Design review of the part built by this model. Coordinates are the model's own, in mm. Face numbers are marked on the shaded views. A direction names the side the tool comes from. Give positions to 0.01 mm unless a question says otherwise; leave off trailing zeros. Loops run counter-clockwise (first coordinate to the right, second up) from the corner with the lowest first, then second, coordinate; pieces in that order, holes last. Notation, with made-up numbers: M 64,-0.5 L 116,-0.5 A26 ccw 116,35.5 Z; hole C 48,-25 d10. An arc over 180 degrees is marked long. Use a Markdown table: item, result. Add a question column.
(1) For the marked faces 1, 2 and 3, list the 3-axis set-ups (+Z, -Z, +X, -X, +Y, -Y) from which the entire face can be reached by the end or side of a thin tool; tool diameter is ignored.
(2) Add section C-C, the plane x = 19.25. Give the boundary of the cut face in (y, z), then the cut area to 3 significant figures.
(3) Add section D-D, the plane z = 48.5. Give the boundary of the cut face in (x, y), then the cut area to 3 significant figures.
(4) Add section A-A, the plane y = -33. Give the boundary of the cut face in (x, z), then the cut area to 3 significant figures.
(5) Insertion check: pin 1 Ø12 at (x, z) = (23.5, 13.5) entering from +Y; pin 2 Ø8 at (x, y) = (19.5, -40.5) entering from -Z; pin 3 Ø4 at (x, y) = (26, -29.5) entering from -Z; pin 4 Ø1.8 at (x, z) = (33.7, 18.8) entering from +Y. Each pin has a flat end and moves straight along its axis. Give the tip position at first contact, or say it passes through.
(6) Add section B-B, the plane z = 18.8. Give the boundary of the cut face in (x, y), then the cut area to 3 significant figures.
(7) Draft analysis for pull direction Z (two halves, no side actions). For the marked faces 4 and 5, state which applies: pulls with the +Z half, pulls with the -Z half, needs draft (parallel to the pull), parting line crosses it, or undercut.
(8) For probe 1 along X at (y, z) = (-27.1, 18.8); probe 2 along Z at (x, y) = (33.7, -27.15); probe 3 along Y at (x, z) = (32, 45), list the stretches that pass through material, from the lowest coordinate up.
```python
from build123d import *

# Parameters (mm, degrees)
SKETCH009_W             = 20
SKETCH009_H             = 35
SKETCH009_R             = 1.5
PAD007_DEPTH            = 2
SKETCH010_R             = 10
PAD008_DEPTH            = 15
SKETCH011_R             = 1.5
PAD009_DEPTH            = 1
SKETCH012_W             = 10
SKETCH012_H             = 2.3
PAD010_DEPTH            = 6
SKETCH013_W             = 10
SKETCH013_H             = 2.3
PAD011_DEPTH            = 11
BODY002_PLACEMENT_ANGLE = 180


with BuildPart() as part:
    # Sketch009 → Pad007 (new body)
    with BuildSketch(Plane.XZ):
        Rectangle(SKETCH009_W, SKETCH009_H)
        with Locations((7.7, 15.2)):
            Circle(SKETCH009_R, mode=Mode.SUBTRACT)
        with Locations((-7.7, 15.2)):
            Circle(SKETCH009_R, mode=Mode.SUBTRACT)
    extrude(amount=PAD007_DEPTH)

    # Sketch010 (on Face8 of Pad007) → Pad008 (join)
    with BuildSketch(Plane.XZ.offset(2)):
        with Locations((0, -6)):
            Circle(SKETCH010_R)
    extrude(amount=PAD008_DEPTH)

    # Sketch011 (on Face4 of Pad008) → Pad009 (join)
    with BuildSketch(Plane(origin=(0, 0, 0), x_dir=(1, 0, 0), z_dir=(0, 1, 0))):
        with Locations((0, 7.5)):
            Circle(SKETCH011_R)
    extrude(amount=PAD009_DEPTH)

    # Sketch012 (on Face5 of Pad009) → Pad010 (join)
    with BuildSketch(Plane.XZ.offset(2)):
        with Locations((0, 15.35)):
            Rectangle(SKETCH012_W, SKETCH012_H)
    extrude(amount=PAD010_DEPTH)

    # Sketch013 (on Face13 of Pad010) → Pad011 (join)
    with BuildSketch(Plane(origin=(0, 0, 16.5), x_dir=(-1, 0, 0), z_dir=(0, 0, 1))):
        with Locations((0, 6.85)):
            Rectangle(SKETCH013_W, SKETCH013_H)
    extrude(amount=PAD011_DEPTH)


with BuildPart() as part_1:
    # Body002 placement: moved
    add(part.part.moved(Location((26, -26, 34))).rotate(Axis((26, -26, 34), (0, 1, 0)), BODY002_PLACEMENT_ANGLE))


solid = part_1.part
```
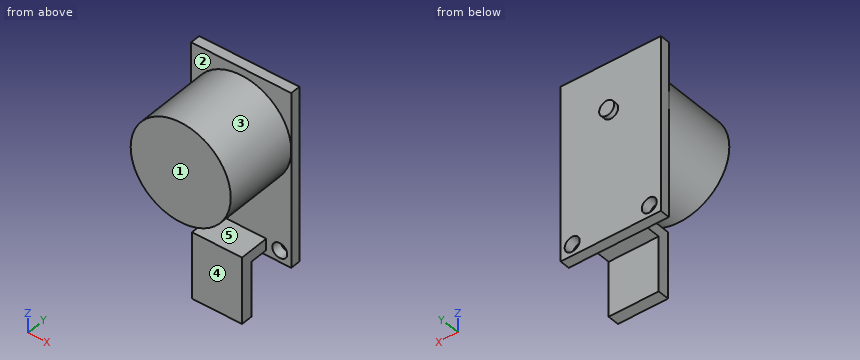
Established:
| question | item | result |
|---|---|---|
| 1 | face 1 | +Z, -Z, +X, -X, -Y |
| 1 | face 2 | +Z, -Y |
| 1 | face 3 | -Y |
| 2 | outline | M -43,32.62 L -28,32.62 L -28,19.96 L -26,19.96 L -26,51.5 L -28,51.5 L -28,47.38 L -43,47.38 Z; M -28,16.5 L -26,16.5 L -26,17.64 L -28,17.64 Z |
| 2 | area | 287 mm^2 |
| 3 | outline | M 16,-28 L 20.73,-28 L 20.73,-43 L 31.27,-43 L 31.27,-28 L 36,-28 L 36,-26 L 16,-26 Z |
| 3 | area | 198 mm^2 |
| 4 | outline | C 26,40 d20; M 21,6.5 L 31,6.5 L 31,19.8 L 21,19.8 Z |
| 4 | area | 447 mm^2 |
| 5 | pin 1 | y = -26 |
| 5 | pin 2 | z = 30.32 |
| 5 | pin 3 | z = 16.5 |
| 5 | pin 4 | through |
| 6 | outline | M 16,-28 L 16.8,-28 L 16.8,-26 L 16,-26 Z; M 19.8,-28 L 21,-28 L 21,-34 L 31,-34 L 31,-28 L 32.2,-28 L 32.2,-26 L 19.8,-26 Z; M 35.2,-28 L 36,-28 L 36,-26 L 35.2,-26 Z |
| 6 | area | 88.0 mm^2 |
| 7 | face 4 | needs draft |
| 7 | face 5 | undercut |
| 8 | probe 1 | 16 to 16.8, 19.8 to 32.2, 35.2 to 36 |
| 8 | probe 2 | 16.5 to 17.3, 20.3 to 51.5 |
| 8 | probe 3 | -43 to -26 |
